from build123d import *

# Parameters (mm, degrees)
CROQUIS1_W              = 798
CROQUIS1_H              = 400
SALIENTE_EXTRUIR1_DEPTH = 50.8
VACIADO1_T              = -1.9
CROQUIS3_R              = 9
CROQUIS3_R_2            = 9.17877309
CORTAR_EXTRUIR1_DEPTH   = 10


with BuildPart() as part:
    # Croquis1 → Saliente-Extruir1 (new body)
    with BuildSketch(Plane(origin=(0, 0, 0), x_dir=(1, 0, 0), z_dir=(0, 1, 0))):
        Rectangle(CROQUIS1_W, CROQUIS1_H)
    extrude(amount=SALIENTE_EXTRUIR1_DEPTH)

    # Vaciado1
    vaciado1_openings = [part.faces().sort_by_distance(p)[0] for p in [
        (0, 0, 0),
    ]]
    offset(amount=VACIADO1_T, openings=vaciado1_openings, kind=Kind.INTERSECTION)

    # Croquis3 → Cortar-Extruir1 (cut)
    with BuildSketch(Plane(origin=(0, 50.8, 0), x_dir=(1, 0, 0), z_dir=(0, 1, 0))):
        with Locations(Location((200, -82.5, 0), (0, 0, 270))):
            Circle(CROQUIS3_R)
        with Locations(Location((200, 168.5, 0), (0, 0, 270))):
            Circle(CROQUIS3_R)
        with Locations(Location((-200, -82.5, 0), (0, 0, 270))):
            Circle(CROQUIS3_R)
        with Locations(Location((-200, 60, 0), (0, 0, 270))):
            Circle(CROQUIS3_R)
        with Locations(Location((-200, 168.5, 0), (0, 0, 270))):
            Circle(CROQUIS3_R_2)
    extrude(amount=-CORTAR_EXTRUIR1_DEPTH, mode=Mode.SUBTRACT)


solid = part.part
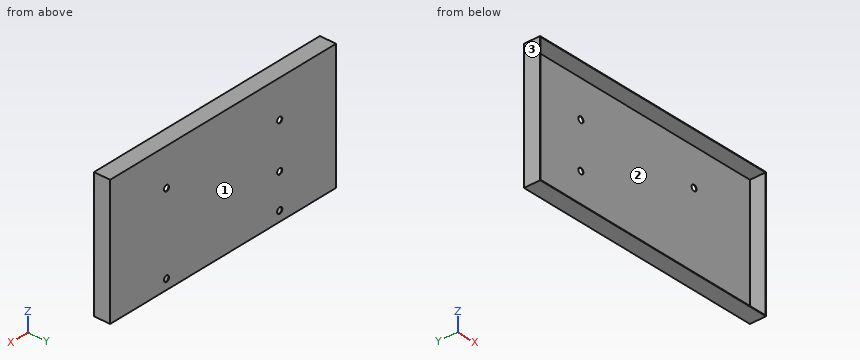
Input: part model. Units: mm. Frame: model coordinates. Face numbers are marked on the shaded views. Coordinates: 2 decimals unless noted, no trailing zeros. Loops run counter-clockwise (first coordinate to the right, second up) from the corner with the lowest first, then second, coordinate; pieces in that order, holes last.
Q1. Cut plane D-D (x = -200). Output: boundary loops of the cut face in (y, z).
Q2. Contact query for a flat-ended pin moving along its axis: pin 1 (4 mm diameter, centred on x = 225, z = 21.5, fed in from -Y). Output: stop coordinate, or through.
Q3. Draft query along X for the marked faces 1, 2 and 3. Return one class per face: +X half, -X half, draft (parallel to the pull), parting line (faces both ways), or undercut.
Q4. Material intervals for line 1 (X direction, y = 49, z = -168); line 2 (X direction, y = 13, z = 116.5); line 3 (Z direction, x = 312, y = 28.5), sorted ascending.
Q5. Cut plane B-B (y = 37). Output: boundary loops of the cut face in (x, z).
Q6. Cut plane C-C (x = 200). Output: boundary loops of the cut face in (y, z), then the cut area to 3 significant figures.
Q7. Cut plane A-A (z = -60). Output: boundary loops of the cut face in (x, y).
Working result:
1. outline: (0, -200) - (50.8, -200) - (50.8, -177.68) - (48.9, -177.68) - (48.9, -198.1) - (0, -198.1) - close; (0, 198.1) - (48.9, 198.1) - (48.9, 91.5) - (50.8, 91.5) - (50.8, 200) - (0, 200) - close; (48.9, -159.32) - (50.8, -159.32) - (50.8, -69) - (48.9, -69) - close; (48.9, -51) - (50.8, -51) - (50.8, 73.5) - (48.9, 73.5) - close
2. pin 1: stops at y = 48.9
3. face 1: draft
3. face 2: undercut
3. face 3: -X half
4. line 1: x = -399 to -209.17, -190.83 to 191.01, 208.99 to 399
4. line 2: x = -399 to -397.1, 397.1 to 399
4. line 3: z = -200 to -198.1, 198.1 to 200
5. outline: (-399, -200) - (399, -200) - (399, 200) - (-399, 200) - close; hole (-397.1, -198.1) - (397.1, -198.1) - (397.1, 198.1) - (-397.1, 198.1) - close
6. outline: (0, -200) - (50.8, -200) - (50.8, -177.5) - (48.9, -177.5) - (48.9, -198.1) - (0, -198.1) - close; (0, 198.1) - (48.9, 198.1) - (48.9, 91.5) - (50.8, 91.5) - (50.8, 200) - (0, 200) - close; (48.9, -159.5) - (50.8, -159.5) - (50.8, 73.5) - (48.9, 73.5) - close
6. area: 877 mm2
7. outline: (-399, 0) - (-397.1, 0) - (-397.1, 48.9) - (-209, 48.9) - (-209, 50.8) - (-399, 50.8) - close; (-191, 48.9) - (397.1, 48.9) - (397.1, 0) - (399, 0) - (399, 50.8) - (-191, 50.8) - close
